```python
from build123d import *

# Parameters (mm, degrees)
F1_DEPTH = 25
F2_DEPTH = 15


with BuildPart() as f1:
    # F0 (on Top) → F1 (new body)
    with BuildSketch(Plane.XY):
        with BuildLine():
            Line((-129.5, -114), (129.5, -114))
            ThreePointArc((129.5, -114), (145.0563491861, -107.5563491861), (151.5, -92))
            Line((151.5, -92), (151.5, 92))
            ThreePointArc((151.5, 92), (145.0563491861, 107.5563491861), (129.5, 114))
            Line((129.5, 114), (-129.5, 114))
            ThreePointArc((-129.5, 114), (-145.0563491861, 107.5563491861), (-151.5, 92))
            Line((-151.5, 92), (-151.5, -92))
            ThreePointArc((-151.5, -92), (-145.0563491861, -107.5563491861), (-129.5, -114))
        make_face()
        with BuildLine():
            ThreePointArc((141.5, -92), (137.9852813742, -100.4852813742), (129.5, -104))
            Line((129.5, -104), (-129.5, -104))
            ThreePointArc((-129.5, -104), (-137.9852813742, -100.4852813742), (-141.5, -92))
            Line((-141.5, -92), (-141.5, 92))
            ThreePointArc((-141.5, 92), (-137.9852813742, 100.4852813742), (-129.5, 104))
            Line((-129.5, 104), (129.5, 104))
            ThreePointArc((129.5, 104), (137.9852813742, 100.4852813742), (141.5, 92))
            Line((141.5, 92), (141.5, -92))
        make_face(mode=Mode.SUBTRACT)
        with BuildLine():
            Line((-129.5, -104), (129.5, -104))
            ThreePointArc((129.5, -104), (137.9852813742, -100.4852813742), (141.5, -92))
            Line((141.5, -92), (141.5, 92))
            ThreePointArc((141.5, 92), (137.9852813742, 100.4852813742), (129.5, 104))
            Line((129.5, 104), (-129.5, 104))
            ThreePointArc((-129.5, 104), (-137.9852813742, 100.4852813742), (-141.5, 92))
            Line((-141.5, 92), (-141.5, -92))
            ThreePointArc((-141.5, -92), (-137.9852813742, -100.4852813742), (-129.5, -104))
        make_face()
    extrude(amount=-F1_DEPTH)

    # F0 (on Top) → F2 (cut)
    with BuildSketch(Plane.XY):
        with BuildLine():
            Line((-129.5, -104), (129.5, -104))
            ThreePointArc((129.5, -104), (137.9852813742, -100.4852813742), (141.5, -92))
            Line((141.5, -92), (141.5, 92))
            ThreePointArc((141.5, 92), (137.9852813742, 100.4852813742), (129.5, 104))
            Line((129.5, 104), (-129.5, 104))
            ThreePointArc((-129.5, 104), (-137.9852813742, 100.4852813742), (-141.5, 92))
            Line((-141.5, 92), (-141.5, -92))
            ThreePointArc((-141.5, -92), (-137.9852813742, -100.4852813742), (-129.5, -104))
        make_face()
    extrude(amount=-F2_DEPTH, mode=Mode.SUBTRACT)


solid = f1.part
```
Can you work these out from the model? Positions are in its coordinate system, mm. A direction names the side the tool comes from. Round coordinates to 2 decimals unless told otherwise and drop trailing zeros. Loops run counter-clockwise (first coordinate to the right, second up) from the corner with the lowest first, then second, coordinate; pieces in that order, holes last. Notation, with made-up numbers: (44, 7) -> (96, 7) arc R24 cw to (96, 27) -> close; hole circle Ø2 at (44, 43). An arc over 180 degrees is marked (long way). Answer in a Markdown table with one row per item.
Item 1: If I drill on probe 1 along X at (y, z) = (3.5, -13.5); probe 2 along Y at (x, z) = (18, -4.5); probe 3 along Z at (x, y) = (123, 59), over which ranges is the centre line in solid material (lowest first)?
Answer block:
| item | result |
|---|---|
| probe 1 | -151.5 to -141.5, 141.5 to 151.5 |
| probe 2 | -114 to -104, 104 to 114 |
| probe 3 | -25 to -15 |
Item 2: Suppose I cut it at A-A, the plane z = -3.5. List the corners of the cut face in (x, y) for me.
Answer block:
| item | result |
|---|---|
| outline | (-151.5, -92) arc R22 ccw to (-129.5, -114) -> (129.5, -114) arc R22 ccw to (151.5, -92) -> (151.5, 92) arc R22 ccw to (129.5, 114) -> (-129.5, 114) arc R22 ccw to (-151.5, 92) -> close; hole (-141.5, -92) arc R12 ccw to (-129.5, -104) -> (129.5, -104) arc R12 ccw to (141.5, -92) -> (141.5, 92) arc R12 ccw to (129.5, 104) -> (-129.5, 104) arc R12 ccw to (-141.5, 92) -> close |
Item 3: Will this pin go through, and if not, where does the flat tip stop? P1, Ø10, axis at x = -15.5, y = -37.5, coming from the +Z side.
Answer block:
| item | result |
|---|---|
| P1 | z = -15 |
Item 4: We'd pull the mould along X, two halves only. Please class faces 1 (the flat face through (-151.5, 1, -12)), 2 (the flat face through (-2, -104, -7)), 3 (the flat face through (2, 114, -12)): released by +X, released by -X, zero draft, split by the parting line, or undercut.
Answer block:
| item | result |
|---|---|
| face 1 | released by -X |
| face 2 | undercut |
| face 3 | zero draft |
Item 5: Suppose I cut it at B-B, the plane x = 95.5. List the corners of the cut face in (y, z) for me.
Answer block:
| item | result |
|---|---|
| outline | (-114, -25) -> (114, -25) -> (114, 0) -> (104, 0) -> (104, -15) -> (-104, -15) -> (-104, 0) -> (-114, 0) -> close |
Item 6: On a 3-axis mill with a long thin cutter (end or side, diameter ignored), from which of +Z, -Z, +X, -X, +Y, -Y can I reach the whole of each face in a straight line? I mean faces 4 (the flat face through (-141.5, 1, -7)), 5 (the cylindrical face through (145.23, 107.38, -12.32)). Say none if no direction works.
Answer block:
| item | result |
|---|---|
| face 4 | +Z |
| face 5 | +Z, -Z, +X, +Y |
Item 7: Suppose I cut it at C-C, the plane y = 77. List the corners of the cut face in (x, z) for me.
Answer block:
| item | result |
|---|---|
| outline | (-151.5, -25) -> (151.5, -25) -> (151.5, 0) -> (141.5, 0) -> (141.5, -15) -> (-141.5, -15) -> (-141.5, 0) -> (-151.5, 0) -> close |
